The listing builds one solid part. Answer for the finished solid, in the listing's coordinates (mm). A direction names the side the tool comes from. Round coordinates to 2 decimals unless told otherwise and drop trailing zeros. Order: outer loops, then holes, each group sorted by start corner. A loop starts at its lowest first (then second) coordinate and runs counter-clockwise, first axis right, second up. Notation, with made-up numbers: (69.25, 81) - (102.25, 81) arc R9 ccw to (102.25, 98) - close; hole circle Ø8 at (50.5, 18.5). An arc over 180 degrees is marked (long way). Write item = value, one per line.
from build123d import *

# Parameters (mm, degrees)
F1_DEPTH       = 127
F2_W           = 711.2
F2_H           = 177.8
F3_DEPTH       = 812.8
F4_D           = 228.6
F4_CSINK_D     = 381
F4_CSINK_ANGLE = 90
F7_DEPTH       = 177.8
F8_DEPTH       = 177.8
F9_D           = 304.8
F11_DEPTH      = 177.8
F13_DEPTH      = 177.8


with BuildPart() as f1:
    # F0 (on Top) → F1 (new body, symmetric)
    with BuildSketch(Plane.XY):
        with BuildLine():
            ThreePointArc((-762, 406.4), (-1168.4, 0), (-762, -406.4))
            Line((-762, -406.4), (762, -406.4))
            ThreePointArc((762, -406.4), (1168.4, 0), (762, 406.4))
            Line((762, 406.4), (-762, 406.4))
        make_face()
    extrude(amount=F1_DEPTH, both=True)

    # F2 (on face) → F3 (join)
    with BuildSketch(Plane.XY.offset(127)):
        with Locations((0, -317.5)):
            Rectangle(F2_W, F2_H)
        with Locations((0, 317.5)):
            Rectangle(F2_W, F2_H)
    extrude(amount=F3_DEPTH)

    # F4 (through all)
    with Locations(Plane.XY.offset(127)):
        with Locations((649.3564248085, 0), (-762, 0)):
            CounterSinkHole(F4_D / 2, F4_CSINK_D / 2, counter_sink_angle=F4_CSINK_ANGLE)

    # F5 (on face) → F7 (cut)
    with BuildSketch(Plane.XZ.offset(406.4)):
        with BuildLine():
            Line((-355.6, 939.8), (-355.6, 584.2))
            ThreePointArc((-355.6, 584.2), (-251.4471708218, 835.6471719581), (1.6069e-06, 939.8))
            Line((1.6069e-06, 939.8), (-355.6, 939.8))
        make_face()
        with BuildLine():
            ThreePointArc((1.6069e-06, 939.8), (251.4471719581, 835.6471708218), (355.6, 584.2))
            Line((355.6, 584.2), (355.6, 939.8))
            Line((355.6, 939.8), (1.6069e-06, 939.8))
        make_face()
    extrude(amount=-F7_DEPTH, mode=Mode.SUBTRACT)

    # F6 (on face) → F8 (cut)
    with BuildSketch(Plane(origin=(0, 406.4, 0), x_dir=(-1, 0, 0), z_dir=(0, 1, 0))):
        with BuildLine():
            Line((-355.6, 939.8), (-355.6, 584.2))
            ThreePointArc((-355.6, 584.2), (-251.4471708218, 835.6471719581), (1.6069e-06, 939.8))
            Line((1.6069e-06, 939.8), (-355.6, 939.8))
        make_face()
        with BuildLine():
            ThreePointArc((1.6069e-06, 939.8), (251.4471719581, 835.6471708218), (355.6, 584.2))
            Line((355.6, 584.2), (355.6, 939.8))
            Line((355.6, 939.8), (1.6069e-06, 939.8))
        make_face()
    extrude(amount=-F8_DEPTH, mode=Mode.SUBTRACT)

    # F9 (through all)
    with Locations(Plane(origin=(0, 406.4, 0), x_dir=(-1, 0, 0), z_dir=(0, 1, 0))):
        with Locations((0, 584.2)):
            Hole(F9_D / 2)

    # F10 (on face) → F11 (join)
    with BuildSketch(Plane.XZ.offset(406.4)):
        with BuildLine():
            Line((-457.2, 127), (-355.6, 127))
            Line((-355.6, 127), (-355.6, 228.6))
            ThreePointArc((-355.6, 228.6), (-385.3579510314, 156.7579510314), (-457.2, 127))
        make_face()
        with BuildLine():
            ThreePointArc((457.2, 127), (385.3579510314, 156.7579510314), (355.6, 228.6))
            Line((355.6, 228.6), (355.6, 127))
            Line((355.6, 127), (457.2, 127))
        make_face()
    extrude(amount=-F11_DEPTH)

    # F12 (on face) → F13 (join)
    with BuildSketch(Plane(origin=(0, 406.4, 0), x_dir=(-1, 0, 0), z_dir=(0, 1, 0))):
        with BuildLine():
            Line((-355.6, 127), (-355.6, 228.6))
            ThreePointArc((-355.6, 228.6), (-385.3579510314, 156.7579510314), (-457.2, 127))
            Line((-457.2, 127), (-355.6, 127))
        make_face()
        with BuildLine():
            ThreePointArc((458.4309247494, 127), (386.5888757808, 156.7579510314), (356.8309247494, 228.6))
            Line((356.8309247494, 228.6), (356.8309247494, 127))
            Line((356.8309247494, 127), (458.4309247494, 127))
        make_face()
    extrude(amount=-F13_DEPTH)


solid = f1.part
Q1. Find the intervals of material crossed by line 1 (X direction, y = 0, z = -82); line 2 (Z direction, x = 0, y = 326.5); line 3 (Y direction, x = -762, z = -46.5), in increasing order. Write a range as from..to.
Model answer:
line_1 = -1168.4..-876.3, -647.7..535.06, 763.66..1168.4
line_2 = -127..431.8, 736.6..939.8
line_3 = -406.4..-114.3, 114.3..406.4
Q2. Section C-C on z = 29 is taken. Determine the outline of the cut face in (x, y).
Model answer:
outline = (-762, -406.4) - (762, -406.4) arc R406.4 ccw to (762, 406.4) - (-762, 406.4) arc R406.4 ccw to start; hole circle Ø228.6 at (-762, 0); hole circle Ø228.6 at (649.36, 0)
Q3. Section B-B on y = 0 is taken. Determine the outline of the cut face in (x, z), then the cut area to 3 significant figures.
Model answer:
outline = (-1168.4, -127) - (-876.3, -127) - (-876.3, 50.8) - (-952.5, 127) - (-1168.4, 127) - close; (-647.7, -127) - (535.06, -127) - (535.06, 50.8) - (458.86, 127) - (-571.5, 127) - (-647.7, 50.8) - close; (763.66, -127) - (1168.4, -127) - (1168.4, 127) - (839.86, 127) - (763.66, 50.8) - close
area = 466,000 mm^2
Q4. Section D-D on y = 314 is taken. Determine the outline of the cut face in (x, z).
Model answer:
outline = (-1020, -127) - (1020, -127) - (1020, 127) - (457.2, 127) arc R101.6 cw to (355.6, 228.6) - (355.6, 584.2) arc R355.6 ccw to (-355.6, 584.2) - (-355.6, 127) - (-356.83, 127) - (-356.83, 228.6) arc R101.6 cw to (-458.43, 127) - (-1020, 127) - close; hole circle Ø304.8 at (0, 584.2)
Q5. Determine the mould class of faces 1 (the face through (-19.839, -318.745, 735.303)), 2 (the face through (-377, 228.6, 152)), 3 (the face through (-1168.3, 8.94, 1.78)) for opening direction Y: released by +Y, released by -Y, zero draft, split by the parting line, or undercut.
Model answer:
face_1 = zero draft
face_2 = undercut
face_3 = split by the parting line
Q6. Section A-A on x = 0 is taken. Determine the outline of the cut face in (y, z).
Model answer:
outline = (-406.4, -127) - (406.4, -127) - (406.4, 431.8) - (228.6, 431.8) - (228.6, 127) - (-228.6, 127) - (-228.6, 431.8) - (-406.4, 431.8) - close; (-406.4, 736.6) - (-228.6, 736.6) - (-228.6, 939.8) - (-406.4, 939.8) - close; (228.6, 736.6) - (406.4, 736.6) - (406.4, 939.8) - (228.6, 939.8) - close
Q7. Flat-ended cylindrical pins translate along their axes: P1, Ø6, axis at x = -930.5, z = 76.5, coming from the +Y side; P2, Ø5, axis at y = 305, z = 184, coming from the +X side; P3, Ø5, axis at x = -9.5, y = 178, coming from the +Z side. Find the tip coordinate at first contact, or state that the pin passes through.
Model answer:
P1 = 371.17
P2 = 367.18
P3 = 127
Q8. For faces 4 (the face through (-7.819, -318.745, 939.714)), 5 (the face through (147, 228.6, 539)), 6 (the face through (355.6, -319, 404)), determine the directions among +Z, -Z, +X, -X, +Y, -Y from which every point of the face is accessible in a straight line to the end or side of a thin tool.
Model answer:
face_4 = +Z, +Y, -Y
face_5 = +Z, +X, -X
face_6 = +Z, +X, +Y, -Y
